```python
from build123d import *

# Parameters (mm, degrees)
BOSS_EXTRUDE1_DEPTH      = 36
BOSS_EXTRUDE1_DEPTH_BACK = 36
FILLET1_R                = 12
M12X1_5_TAPPED_HOLE1_D   = 10.5


with BuildPart() as part:
    # Sketch1 → Boss-Extrude1 (new, two sides: drawn at the far end of the back side and taken through both)
    with BuildSketch(Plane.XY.offset(-BOSS_EXTRUDE1_DEPTH_BACK)):
        Polygon((-25, 8), (-25, 5), (0, 5), (25, 5), (25, 8), (0, 8), align=None)
        Polygon((0, 5), (-25, 5), (-60, 5), (-60, -5), (-28, -5), (-25, -2), (0, -2), align=None)
        Polygon((25, 5), (0, 5), (0, -2), (25, -2), (28, -5), (60, -5), (60, 5), align=None)
    extrude(amount=BOSS_EXTRUDE1_DEPTH + BOSS_EXTRUDE1_DEPTH_BACK)

    # Fillet1
    fillet1_edges = [part.edges().sort_by_distance(p)[0] for p in [
        (-60, 0, -36),
        (60, 0, 36),
        (-60, 0, 36),
        (60, 0, -36),
    ]]
    fillet(fillet1_edges, radius=FILLET1_R)

    # M12x1.5 Tapped Hole1 (through all)
    with Locations(Plane(origin=(0, 5, 0), x_dir=(1, 0, 0), z_dir=(0, 1, 0))):
        with Locations((-48, -24), (-48, 24), (48, 24), (48, -24)):
            Hole(M12X1_5_TAPPED_HOLE1_D / 2)


solid = part.part
```
For this review, take the finished solid that the model builds, in its own axes (mm). A direction names the side the tool comes from. Coordinates: 2 decimals unless noted, no trailing zeros. Loops run counter-clockwise (first coordinate to the right, second up) from the corner with the lowest first, then second, coordinate; pieces in that order, holes last. Notation, with made-up numbers: (-19.75, -30) - (10.25, -30) arc R9 ccw to (10.25, -16) - close; hole circle Ø5 at (-24, 10.25). An arc over 180 degrees is marked (long way). Use one line per item in the form item = value. Start each with the question number.
1) Draft analysis for pull direction X (two halves, no side actions). For faces 1 (the face through (-27, -4, -1)), 2 (the face through (0, 8, -1)), 3 (the face through (60, 0, 0)), 4 (the face through (-43.83, -0.07, -20.81)), state which applies: released by +X, released by -X, zero draft, split by the parting line, or undercut.
2) To check wall thickness, follow probe 1 along Z at (x, y) = (48, 2.5); probe 2 along X at (y, z) = (2.75, -24); probe 3 along X at (y, z) = (2.25, -20.5). State the ranges of each line that lie inside material, in increasing order. Write a range as from..to.
3) Take a section at D-D (x = -12.5). State the section outline as (y, z) points, plus the area to 3 significant figures.
4) Take a section at B-B (z = -4.5). State the section outline as (x, y) points, plus the area to 3 significant figures.
5) Take a section at C-C (z = 21). State the section outline as (x, y) points, plus the area to 3 significant figures.
6) For pin 1 (0.9 mm diameter, centred on y = 6, z = 15, fed in from +X); pin 2 (6.5 mm diameter, centred on x = 48, z = -24, fed in from +Y); pin 3 (0.9 mm diameter, centred on y = 7, z = -1.5, fed in from -X); pin 4 (10.5 mm diameter, centred on x = -40, z = 15, fed in from +Y), all flat-tipped, find the tip position at first contact; note any pin that passes through.
7) Take a section at A-A (y = 2.25). State the section outline as (x, z) points.
8) For faces 5 (the face through (-25, 7, -1)), 6 (the face through (43, 5, -1)), 7 (the face through (26, -3, -1)), 8 (the face through (56.58, 0.07, -32.39)), list the 3-axis set-ups (+Z, -Z, +X, -X, +Y, -Y) from which the entire face can be reached by the end or side of a thin tool; tool diameter is ignored.
From the geometry:
q1.face_1 = undercut
q1.face_2 = zero draft
q1.face_3 = released by +X
q1.face_4 = undercut
q2.probe_1 = -36..-29.25, -18.75..18.75, 29.25..36
q2.probe_2 = -60..-53.25, -42.75..42.75, 53.25..60
q2.probe_3 = -60..-51.91, -44.09..44.09, 51.91..60
q3.outline = (-2, -36) - (8, -36) - (8, 36) - (-2, 36) - close
q3.area = 720 mm2
q4.outline = (-60, -5) - (-28, -5) - (-25, -2) - (25, -2) - (28, -5) - (60, -5) - (60, 5) - (25, 5) - (25, 8) - (-25, 8) - (-25, 5) - (-60, 5) - close
q4.area = 1,190 mm2
q5.outline = (-60, -5) - (-52.31, -5) - (-52.31, 5) - (-60, 5) - close; (-43.69, -5) - (-28, -5) - (-25, -2) - (25, -2) - (28, -5) - (43.69, -5) - (43.69, 5) - (25, 5) - (25, 8) - (-25, 8) - (-25, 5) - (-43.69, 5) - close; (52.31, -5) - (60, -5) - (60, 5) - (52.31, 5) - close
q5.area = 1,020 mm2
q6.pin_1 = 25
q6.pin_2 = through
q6.pin_3 = -25
q6.pin_4 = 5
q7.outline = (-60, -24) arc R12 ccw to (-48, -36) - (48, -36) arc R12 ccw to (60, -24) - (60, 24) arc R12 ccw to (48, 36) - (-48, 36) arc R12 ccw to (-60, 24) - close; hole circle Ø10.5 at (-48, -24); hole circle Ø10.5 at (-48, 24); hole circle Ø10.5 at (48, -24); hole circle Ø10.5 at (48, 24)
q8.face_5 = +Z, -Z, -X, +Y
q8.face_6 = +Z, -Z, +X, +Y
q8.face_7 = +Z, -Z, -Y
q8.face_8 = -Z, +X, +Y, -Y
